Model file for the job. Use its own axes, mm. Face numbers are marked on the shaded views. A direction names the side the tool comes from. Coordinates: 2 decimals unless noted, no trailing zeros. Order: outer loops, then holes, each group sorted by start corner. A loop starts at its lowest first (then second) coordinate and runs counter-clockwise, first axis right, second up. Notation, with made-up numbers: M -28.5,3.25 L -13.5,3.25 A31 ccw -13.5,36.25 Z; hole C -33,83.25 d2. An arc over 180 degrees is marked long. Return JSON: item names as keys, results as strings.
```python
from build123d import *

# Parameters (mm, degrees)
ESQUISSE1_W                = 45
ESQUISSE1_H                = 19
BOSS_EXTRU_1_DEPTH         = 3
R_P_TITION_LIN_AIRE3_COUNT = 2
R_P_TITION_LIN_AIRE3_PITCH = 32
ESQUISSE7_W                = 15.8
ESQUISSE7_H                = 5
BOSS_EXTRU_2_DEPTH         = 45
ESQUISSE8_W                = 29
ESQUISSE8_H                = 12.8
ENL_V_MAT_EXTRU_4_DEPTH    = 3
ESQUISSE8_5_W              = 29
ESQUISSE8_5_H              = 12.8
ENL_V_MAT_EXTRU_5_DEPTH    = 6
ESQUISSE9_R                = 2.3
ENL_V_MAT_EXTRU_6_DEPTH    = 10


with BuildPart() as part:
    # Esquisse1 → Boss.-Extru.1 (new body)
    with BuildSketch(Plane.XY):
        with Locations((22.5, 9.5)):
            Rectangle(ESQUISSE1_W, ESQUISSE1_H)
    extrude(amount=BOSS_EXTRU_1_DEPTH)

    # Esquisse5 → Fraisage pour vis _ t_te frais_e M42 (revolve, cut)
    with BuildSketch(Plane(origin=(38.5, 10.1, 3), x_dir=(0, -1, 0), z_dir=(1, 0, 0))):
        Polygon((0, 0), (0, 3), (2.25, 3), (2.25, 2.45), (4.7, 0), align=None)
    fraisage_pour_vis_t_te_frais_e_m42 = revolve(axis=Axis((38.5, 10.1, 9.35), (0, 0, -1)), mode=Mode.SUBTRACT)

    # R_p_tition lin_aire3: Fraisage pour vis _ t_te frais_e M42 ×2
    with Locations(*[(-i * R_P_TITION_LIN_AIRE3_PITCH, 0, 0) for i in range(1, R_P_TITION_LIN_AIRE3_COUNT)]):
        add(fraisage_pour_vis_t_te_frais_e_m42, mode=Mode.SUBTRACT)

    # Esquisse7 → Boss.-Extru.2 (add)
    with BuildSketch(Plane(origin=(45, 19, 0), x_dir=(0, 0, 1), z_dir=(-1, 0, 0))):
        with Locations((7.9, 2.5)):
            Rectangle(ESQUISSE7_W, ESQUISSE7_H)
    extrude(amount=BOSS_EXTRU_2_DEPTH)

    # Esquisse8 → Enl_v. mat.-Extru.4 (cut)
    with BuildSketch(Plane.XZ.offset(-19)):
        with Locations((22.5, 9.4)):
            Rectangle(ESQUISSE8_W, ESQUISSE8_H)
    extrude(amount=-ENL_V_MAT_EXTRU_4_DEPTH, mode=Mode.SUBTRACT)

    # Esquisse8_5 → Enl_v. mat.-Extru.5 (cut, through all)
    with BuildSketch(Plane.XZ.offset(-19)):
        with Locations((22.5, 9.4)):
            Rectangle(ESQUISSE8_5_W, ESQUISSE8_5_H)
    extrude(amount=-ENL_V_MAT_EXTRU_5_DEPTH, mode=Mode.SUBTRACT)

    # Esquisse9 → Enl_v. mat.-Extru.6 (cut)
    with BuildSketch(Plane(origin=(0, 24, 0), x_dir=(1, 0, 0), z_dir=(0, 1, 0))):
        with Locations((40.3, -9.1)):
            Circle(ESQUISSE9_R)
    enl_v_mat_extru_6 = extrude(amount=-ENL_V_MAT_EXTRU_6_DEPTH, mode=Mode.SUBTRACT)

    # Sym_trie1: Enl_v. mat.-Extru.6 across plane
    add(enl_v_mat_extru_6.mirror(Plane(origin=(22.5, 0, 0), x_dir=(0, 0, 1), z_dir=(1, 0, 0))), mode=Mode.SUBTRACT)


solid = part.part
```
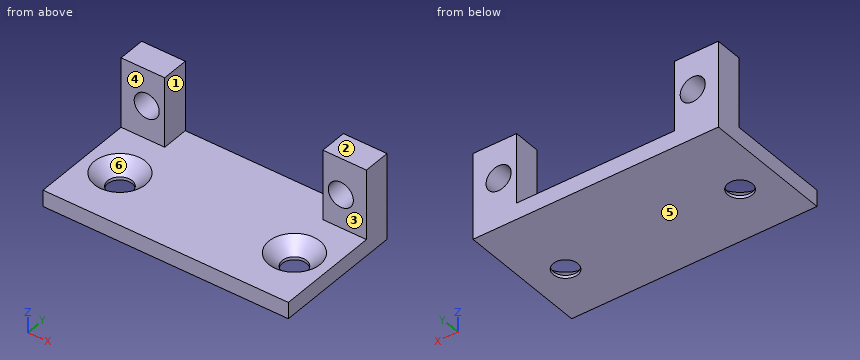
Item 1: Drop flat-ended pins along their axis: pin 1 Ø4 at (x, z) = (41.5, 11.5) entering from -Y; pin 2 Ø4 at (x, y) = (17.5, 13.5) entering from +Z. Give the stop position or say it passes through.
Check result:
{"pin 1": "stops at y = 19", "pin 2": "stops at z = 3"}
Item 2: Wall check: line 1 (X direction, y = 21.4, z = 9.1); line 2 (X direction, y = 10.1, z = 0.1); line 3 (X direction, y = 22, z = 3.25). Give the ranges that are in metal, low to high.
Check result:
{"line 1": "x = 0 to 2.4, 7 to 8, 37 to 38, 42.6 to 45", "line 2": "x = 0 to 4.25, 8.75 to 36.25, 40.75 to 45", "line 3": "x = 0 to 8, 37 to 45"}
Item 3: Saw through at D-D (y = 22.5). Write the cut outline in (x, z), and give its area (3 significant figures).
Check result:
{"outline": "M 0,0 L 45,0 L 45,15.8 L 37,15.8 L 37,3 L 8,3 L 8,15.8 L 0,15.8 Z; hole C 4.7,9.1 d4.6; hole C 40.3,9.1 d4.6", "area": "307 mm2"}
Item 4: Pull direction Y, two halves, no side cores. Call the marked faces 4, 5 and 6: +Y half, -Y half, draft (parallel to the pull), parting line (faces both ways), or undercut.
Check result:
{"face 4": "-Y half", "face 5": "draft", "face 6": "undercut"}
Item 5: Saw through at C-C (z = 4.25). Write the cut outline in (x, y), and give its area (3 significant figures).
Check result:
{"outline": "M 0,19 L 8,19 L 8,24 L 0,24 Z; M 37,19 L 45,19 L 45,24 L 37,24 Z", "area": "80.0 mm2"}
Item 6: Saw through at A-A (z = 9.1). Write the cut outline in (x, y).
Check result:
{"outline": "M 0,19 L 2.4,19 L 2.4,24 L 0,24 Z; M 7,19 L 8,19 L 8,24 L 7,24 Z; M 37,19 L 38,19 L 38,24 L 37,24 Z; M 42.6,19 L 45,19 L 45,24 L 42.6,24 Z"}
Item 7: Saw through at B-B (y = 10.1). Write the cut outline in (x, z).
Check result:
{"outline": "M 0,0 L 4.25,0 L 4.25,0.55 L 1.8,3 L 0,3 Z; M 8.75,0 L 36.25,0 L 36.25,0.55 L 33.8,3 L 11.2,3 L 8.75,0.55 Z; M 40.75,0 L 45,0 L 45,3 L 43.2,3 L 40.75,0.55 Z"}
Item 8: 3-axis set-ups, long thin cutter, end or side, ignore diameter. For the marked faces 1, 2 and 3: which of +Z, -Z, +X, -X, +Y, -Y reach the whole face in a straight line?
Check result:
{"face 1": "+Z, +Y, -Y", "face 2": "+Z, +X, -X, +Y, -Y", "face 3": "+Z, +X, -X, -Y"}
